from build123d import *

# Parameters (mm, degrees)
SKETCH1_R           = 1.5875
EXTRUDE1_DEPTH      = 9.525
SKETCH2_R           = 3.175
EXTRUDE2_DEPTH      = 1.5875
CHAMFER1_SIZE       = 0.3175
EXTRUDE3_DEPTH      = 12.985362166
EXTRUDE3_DEPTH_BACK = 12.985362166
SKETCH3_R           = 1.190625
CHAMFER2_SIZE       = 0.15875


with BuildPart() as part:
    # Sketch1 → Extrude1 (new, symmetric)
    with BuildSketch(Plane.XY):
        with Locations(Location((0, 0, 0), (0, 0, 180))):
            Circle(SKETCH1_R)
    extrude(amount=EXTRUDE1_DEPTH, both=True)

    # Sketch2 → Extrude2 (add)
    with BuildSketch(Plane.XY.offset(9.525)):
        Circle(SKETCH2_R)
    extrude(amount=EXTRUDE2_DEPTH)

    # Chamfer1
    chamfer1_edges = [part.edges().sort_by_distance(p)[0] for p in [
        (-3.175, 0, 11.1125),
    ]]
    chamfer(chamfer1_edges, length=CHAMFER1_SIZE)

    # Sketch3 → Extrude3 (cut, two sides: drawn at the far end of the back side and taken through both)
    with BuildSketch(Plane(origin=(0, 0, 0), x_dir=(0, 0, -1), z_dir=(1, 0, 0)).offset(-EXTRUDE3_DEPTH_BACK)):
        with Locations(Location((5.953125, 0, 0), (0, 0, 180))):
            Circle(SKETCH3_R)
    extrude(amount=EXTRUDE3_DEPTH + EXTRUDE3_DEPTH_BACK, mode=Mode.SUBTRACT)

    # Chamfer2
    chamfer2_edges = [part.edges().sort_by_distance(p)[0] for p in [
        (1.5875, 0, -9.525),
    ]]
    chamfer(chamfer2_edges, length=CHAMFER2_SIZE)


solid = part.part
Can you work these out from the model? Positions are in its coordinate system, mm. A direction names the side the tool comes from. Coordinates: 2 decimals unless noted, no trailing zeros. Loops run counter-clockwise (first coordinate to the right, second up) from the corner with the lowest first, then second, coordinate; pieces in that order, holes last. Notation, with made-up numbers: (-2, 30.25) - (20, 30.25) arc R6 ccw to (20, 34.25) - close; hole circle Ø3 at (19, 61). An arc over 180 degrees is marked (long way). Answer as a JSON object with one key per item and string values. Group by question number.
Item 1: On a 3-axis mill with a long thin cutter (end or side, diameter ignored), from which of +Z, -Z, +X, -X, +Y, -Y can I reach the whole of each face in a straight line? I mean faces 1 (the face through (0, 0, -9.525)), 2 (the face through (-1.514, -0.477, 0.212)). Say none if no direction works.
Item 2: For pin 1 (1.5 mm diameter, centred on y = 0.5, z = -3, fed in from -X); pin 2 (2 mm diameter, centred on x = 1.5, z = 0.5, fed in from -Y); pin 3 (3 mm diameter, centred on y = 0, z = -5.95, fed in from +X), each with a flat end and sliding along its axis, tell me the tip position at first contact or that it passes through.
Item 3: If we section it at C-C (z = 0.5): List the corners of the cut face in (x, y) for me (1 decimal), plus the area to 3 significant figures.
Item 4: If I drill on L1, parallel to Y at x = 0, z = -4.5; L2, parallel to Z at x = -2.25, y = 0.25 (1 decimal); L3, parallel to Z at x = -0.25, y = -1 (1 decimal), over which ranges is the centre line in solid material (lowest first)? Write a range as from..to.
Item 5: If we mould it in two halves opening along Z, with no side actions, what happens to faces 3 (the face through (-0.02, 1.056, -5.404)), 4 (the face through (0, 0, 11.112)), 5 (the face through (1.4, -1.4, 9.525))? For each: released by +Z, released by -Z, zero draft, split by the parting line, or undercut.
Returned:
{
 "1": {"face 1": "-Z, +X, -X, +Y, -Y", "face 2": "-Z"},
 "2": {"pin 1": "stops at x = -1.59", "pin 2": "stops at y = -1.51", "pin 3": "stops at x = 1.59"},
 "3": {"outline": "circle Ø3.2 at (0, 0)", "area": "7.92 mm²"},
 "4": {"L1": "y = -1.59..1.59", "L2": "z = 9.5..11.1", "L3": "z = -9.5..-6.6, -5.3..11.1"},
 "5": {"face 3": "undercut", "face 4": "released by +Z", "face 5": "released by -Z"}
}
